from build123d import *

# Parameters (mm, degrees)
F0_W     = 173.918859
F0_H     = 254
F1_DEPTH = 25.4
F3_D     = 25.4
F5_D     = 25.4


with BuildPart() as f1:
    # F0 (on Right) → F1 (new body)
    with BuildSketch(Plane.YZ):
        with Locations((-22.266922, -7.02697)):
            Rectangle(F0_W, F0_H)
    extrude(amount=F1_DEPTH)

    # F3 (through all)
    with Locations(Plane(origin=(0, 0, 0), x_dir=(0, -1, 0), z_dir=(-1, 0, 0))):
        with Locations((-21.514764, -81.443645), (72.651654, -81.443645), (-21.514764, 75.946935), (72.651654, 75.946935)):
            Hole(F3_D / 2)

    # F5 (through all)
    with Locations(Plane(origin=(0, 0, 0), x_dir=(0, -1, 0), z_dir=(-1, 0, 0))):
        with Locations((84.372841, -55.81788), (84.372841, 42.938467)):
            Hole(F5_D / 2)


solid = f1.part
Source: CAD feature listing. Evaluate the final solid. Frame: model axes, mm. Give positions to 0.01 mm unless a question says otherwise; leave off trailing zeros. Loops run counter-clockwise (first coordinate to the right, second up) from the corner with the lowest first, then second, coordinate; pieces in that order, holes last. Notation, with made-up numbers: (-8.5, -6) -> (13.5, -6) arc R21 cw to (13.5, -1) -> close; hole circle Ø3 at (74.5, -1.75). An arc over 180 degrees is marked (long way). Use a Markdown table: item, result. Add a question column.
1) Line query: line 1 along Z through (x, y) = (23.25, -68.5); line 2 along Y through (x, z) = (22.25, 69); line 3 along Z through (x, y) = (14.25, -89). Output: solid intervals per line, ascending. Write a range as [from, to].
2) Section query A-A, the plane y = -91.5. Return the cut outline in (x, z), then the cut area to 3 significant figures.
3) Pull-direction query (Z, two-part tool) for faces 1 (the face through (12.878, -75.405, 63.549)), 2 (the face through (13, -23, -134.027)), 3 (the face through (0, -23, -5)), 4 (the face through (13, -23, 119.973)); classes: +Z half, -Z half, draft (parallel to the pull), parting line (faces both ways), or undercut.
4) Section query C-C, the plane x = 7. Return the cut outline in (y, z), then the cut area to 3 significant figures.
5) Section query B-B, the plane z = -75.5. Return the cut outline in (x, y).
Numbers:
| question | item | result |
|---|---|---|
| 1 | line 1 | z = [-134.03, -93.45], [-69.44, 63.94], [87.95, 119.97] |
| 1 | line 2 | y = [-109.23, -83.28], [-62.02, 10.88], [32.15, 64.69] |
| 1 | line 3 | z = [-134.03, -67.64], [-43.99, 31.11], [54.77, 119.97] |
| 2 | outline | (0, -134.03) -> (25.4, -134.03) -> (25.4, -66.33) -> (0, -66.33) -> close; (0, -45.31) -> (25.4, -45.31) -> (25.4, 32.43) -> (0, 32.43) -> close; (0, 53.45) -> (25.4, 53.45) -> (25.4, 119.97) -> (0, 119.97) -> close |
| 2 | area | 5,380 mm2 |
| 3 | face 1 | undercut |
| 3 | face 2 | -Z half |
| 3 | face 3 | draft |
| 3 | face 4 | +Z half |
| 4 | outline | (-109.23, -134.03) -> (64.69, -134.03) -> (64.69, 119.97) -> (-109.23, 119.97) -> close; hole circle Ø25.4 at (-84.37, -55.82); hole circle Ø25.4 at (-84.37, 42.94); hole circle Ø25.4 at (-72.65, -81.44); hole circle Ø25.4 at (-72.65, 75.95); hole circle Ø25.4 at (21.51, -81.44); hole circle Ø25.4 at (21.51, 75.95) |
| 4 | area | 41,100 mm2 |
| 5 | outline | (0, -109.23) -> (25.4, -109.23) -> (25.4, -83.87) -> (0, -83.87) -> close; (0, -61.43) -> (25.4, -61.43) -> (25.4, 10.29) -> (0, 10.29) -> close; (0, 32.74) -> (25.4, 32.74) -> (25.4, 64.69) -> (0, 64.69) -> close |
